Design review of the part built by this model. Coordinates are the model's own, in mm. Give positions to 0.01 mm unless a question says otherwise; leave off trailing zeros. Write each loop counter-clockwise with the first axis right and the second up, starting at its lowest first coordinate (ties: lowest second). Pieces come first, ordered by that corner, then holes. Notation, with made-up numbers: (7, 55) -> (16, 55) arc R9 cw to (16, 62) -> close; hole circle Ø10 at (19, 87.5). An arc over 180 degrees is marked (long way). Answer as a JSON object with one key per item and string values.
Autodesk Inventor part; units mm, degrees
ref_plane "YZ Plane" through (0, 0, 0) normal (1, 0, 0) x (0, 1, 0)
ref_plane "XZ Plane" through (0, 0, 0) normal (0, 1, 0) x (-1, 0, 0)
ref_plane "XY Plane" through (0, 0, 0) normal (0, 0, 1) x (1, 0, 0)
sketch "Sketch1" plane through (0, 0, 0) normal (1, 0, 0) x (0, 1, 0)
  circle A0 centre (0, 0) radius 21
  line L0 (36, -46) -> (36, 34)
  line L1 (36, 34) -> (-29, 34)
  line L2 (-29, 34) -> (-29, -46)
  line L3 (-29, -46) -> (36, -46)
  point P0 (0, -17.5)
  point P1 (17.5, 0)
  point P2 (0, 17.5)
  point P3 (-17.5, 0)
  point P4 (0, -30)
  point P5 (0, 30)
  point P6 (31, -41)
  point P7 (31, 29)
  point P8 (-24, 29)
  point P9 (-24, -41)
  dimension "d6" = 30
  dimension "d9" = 360
  dimension "d15" = 5
  dimension "d16" = 5
  dimension "d17" = 80
  dimension "d18" = 65
  dimension "d28" = 5
  dimension "d29" = 55
  dimension "d30" = 55
  dimension "d38" = 42
extrude "Extrusion1" add sketch "Sketch1" along normal blind 2
hole "Hole1" at (0, 0, -17.5) at (0, 17.5, 0) at (0, 0, 17.5) at (0, -17.5, 0) at (0, 31, -41) at (0, 31, 29) at (0, -24, 29) at (0, -24, -41) direction (1, 0, 0) diameter 3.2 depth 43.75 tip angle 118
sketch "Sketch2" plane through (0, 0, 0) normal (-1, 0, 0) x (0, 0, 1)
  circle A0 centre (-40, 0) radius 6
  line L0 (-46, 36) -> (34, 36)
  line L1 (-46, 36) -> (-52, 36)
  line L2 (-52, 36) -> (-52, -29)
  line L3 (-52, -29) -> (-46, -29)
  line L4 (-46, -29) -> (-46, 36)
  point P0 (0, 0)
  point P1 (0, 25.1294)
  point P2 (0, -32.6005)
  dimension "d31" = 40
  dimension "d32" = 12
  dimension "d33" = 6
extrude "Extrusion2" add sketch "Sketch2" against normal blind 2 contours L4 L3 L2 L1
extrude "Extrusion3" cut sketch "Sketch2" against normal blind 2 contours A0
sketch "Sketch3" plane through (2, 0, 0) normal (1, 0, 0) x (0, 0, -1)
  circle A0 centre (-29, 31) radius 1.6
  circle A1 centre (41, 31) radius 1.6
  point P0 (0, 0)
  point P1 (-19, 31)
  point P2 (31, 31)
  point P3 (-19, -24)
  point P4 (31, -24)
  dimension "d39" = 10
  dimension "d40" = 10
hole "Hole2" at (2, 31, 19) at (2, 31, -31) at (2, -24, 19) at (2, -24, -31) direction (-1, 0, 0) diameter 3.2 depth 43.75 tip angle 118
fillet "Fillet1" radius 2 4 edges at (1, 36, 34) (1, 36, -52) (1, -29, -52) (1, -29, 34)
properties part number "motor" material "アルミニウム 6061"
(1) We need section D-D, the plane z = 29. State the section outline as (x, y) points, then the cut area to 3 significant figures.
Here are the results:
{"outline": "(0, -29) -> (2, -29) -> (2, -25.6) -> (0, -25.6) -> close; (0, -22.4) -> (2, -22.4) -> (2, 29.4) -> (0, 29.4) -> close; (0, 32.6) -> (2, 32.6) -> (2, 36) -> (0, 36) -> close", "area": "117 mm²"}
(2) We need section B-B, the plane x = 1.25. Give the number of separate pieces and of enclosed holes in the cut face, then the cut area to 3 significant figures.
Here are the results:
{"separate pieces": "1", "enclosed holes": "10", "area": "4,020 mm²"}
(3) We need section C-C, the plane y = 0. State the section outline as (x, z) points.
Here are the results:
{"outline": "(0, -52) -> (2, -52) -> (2, -46) -> (0, -46) -> close; (0, -34) -> (2, -34) -> (2, -21) -> (0, -21) -> close; (0, 21) -> (2, 21) -> (2, 34) -> (0, 34) -> close"}
(4) For line 1 along Y through (x, z) = (0.65, 29); line 2 along Z through (x, y) = (0.9, -24); line 3 along Z through (x, y) = (1.25, 0), list the stretches that pass through material, from the lowest coordinate up.
Here are the results:
{"line 1": "y = -29 to -25.6, -22.4 to 29.4, 32.6 to 36", "line 2": "z = -52 to -42.6, -39.4 to -32.6, -29.4 to 17.4, 20.6 to 27.4, 30.6 to 34", "line 3": "z = -52 to -46, -34 to -21, 21 to 34"}
(5) We need section A-A, the plane y = 31. State the section outline as (x, z) points, then the cut area to 3 significant figures.
Here are the results:
{"outline": "(0, -52) -> (2, -52) -> (2, -42.6) -> (0, -42.6) -> close; (0, -39.4) -> (2, -39.4) -> (2, -32.6) -> (0, -32.6) -> close; (0, -29.4) -> (2, -29.4) -> (2, 17.4) -> (0, 17.4) -> close; (0, 20.6) -> (2, 20.6) -> (2, 27.4) -> (0, 27.4) -> close; (0, 30.6) -> (2, 30.6) -> (2, 34) -> (0, 34) -> close", "area": "146 mm²"}
(6) The part is to be moulded in two halves that separate along Y. For faces 1 (the cylindrical face through (1.01, 35.43, 33.4)), 2 (the cylindrical face through (1.01, -28.43, -51.4)), 3 (the cylindrical face through (0.99, -25.08, 20.18)), say which applies: +Y half, -Y half, draft (parallel to the pull), parting line (faces both ways), or undercut.
Here are the results:
{"face 1": "+Y half", "face 2": "-Y half", "face 3": "undercut"}
